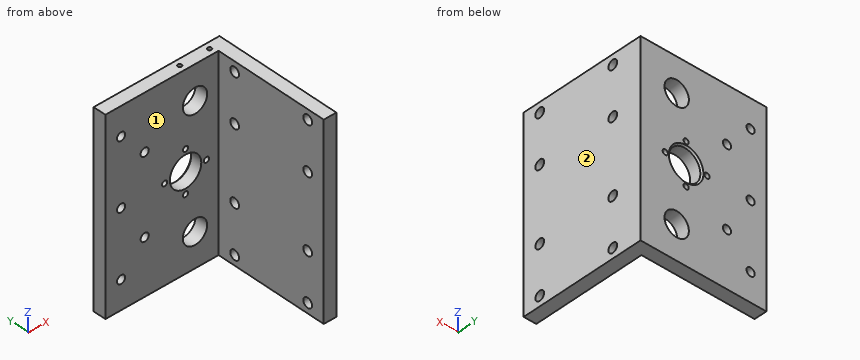
from build123d import *

# Parameters (mm, degrees)
ESTRUSIONE_ESTRUSIONE1_DEPTH = 120
TAGLIO_ESTRUSIONE2_REACH     = 82
SCHIZZO6_R                   = 7.75
TAGLIO_ESTRUSIONE3_REACH     = 82
SCHIZZO7_R                   = 10
M4_TAPPED_HOLE1_D            = 3.3
SCHIZZO12_R                  = 3
TAGLIO_ESTRUSIONE4_DEPTH     = 10
SCHIZZO14_R                  = 2.6
TAGLIO_ESTRUSIONE5_DEPTH     = 10
SMUSSO2_SIZE                 = 1
FORO_FILETTATO_M3_1_D        = 2.5
FORO_FILETTATO_M3_1_DEPTH    = 10
FORO_FILETTATO_M3_1_TIP      = 0.751075774


with BuildPart() as part:
    # Schizzo1 → Estrusione-Estrusione1 (new body)
    with BuildSketch(Plane.XY):
        Polygon((0, 0), (-80, 0), (-80, -8), (-8, -8), (-8, -80), (0, -80), align=None)
    extrude(amount=ESTRUSIONE_ESTRUSIONE1_DEPTH)

    # Schizzo6 → Taglio-Estrusione2 (cut, up to next)
    with BuildSketch(Plane(origin=(0, 0, 0), x_dir=(1, 0, 0), z_dir=(0, 1, 0)), mode=Mode.PRIVATE) as taglio_estrusione2_sk1:
        with Locations((-23, -21.5)):
            Circle(SCHIZZO6_R)
    taglio_estrusione2_tool1 = extrude(taglio_estrusione2_sk1.sketch, amount=-TAGLIO_ESTRUSIONE2_REACH, mode=Mode.PRIVATE) & part.part
    add(taglio_estrusione2_tool1.solids().sort_by_distance((-23, 0, 21.5))[0], mode=Mode.SUBTRACT)
    # Schizzo6 → Taglio-Estrusione2 (cut, up to next)
    with BuildSketch(Plane(origin=(0, 0, 0), x_dir=(1, 0, 0), z_dir=(0, 1, 0)), mode=Mode.PRIVATE) as taglio_estrusione2_sk2:
        with Locations((-23, -98.5)):
            Circle(SCHIZZO6_R)
    taglio_estrusione2_tool2 = extrude(taglio_estrusione2_sk2.sketch, amount=-TAGLIO_ESTRUSIONE2_REACH, mode=Mode.PRIVATE) & part.part
    add(taglio_estrusione2_tool2.solids().sort_by_distance((-23, 0, 98.5))[0], mode=Mode.SUBTRACT)

    # Schizzo7 → Taglio-Estrusione3 (cut, up to next)
    with BuildSketch(Plane(origin=(0, 0, 0), x_dir=(1, 0, 0), z_dir=(0, 1, 0)), mode=Mode.PRIVATE) as taglio_estrusione3_sk1:
        with Locations((-29, -60)):
            Circle(SCHIZZO7_R)
    taglio_estrusione3_tool1 = extrude(taglio_estrusione3_sk1.sketch, amount=-TAGLIO_ESTRUSIONE3_REACH, mode=Mode.PRIVATE) & part.part
    add(taglio_estrusione3_tool1.solids().sort_by_distance((-29, 0, 60))[0], mode=Mode.SUBTRACT)

    # M4 Tapped Hole1 (through all)
    with Locations(Plane(origin=(0, 0, 0), x_dir=(1, 0, 0), z_dir=(0, 1, 0))):
        with Locations((-29, -46.7), (-42.3, -60), (-29, -73.3), (-15.7, -60), (-29, -60)):
            Hole(M4_TAPPED_HOLE1_D / 2)

    # Schizzo12 → Taglio-Estrusione4 (cut)
    with BuildSketch(Plane(origin=(0, 0, 0), x_dir=(0, 0, -1), z_dir=(1, 0, 0))):
        with Locations((-113.75, -19)):
            Circle(SCHIZZO12_R)
        with Locations((-83.25, -19)):
            Circle(SCHIZZO12_R)
        with Locations((-36.75, -19)):
            Circle(SCHIZZO12_R)
        with Locations((-6.25, -19)):
            Circle(SCHIZZO12_R)
        with Locations((-83.25, -69)):
            Circle(SCHIZZO12_R)
        with Locations((-113.75, -69)):
            Circle(SCHIZZO12_R)
        with Locations((-6.25, -69)):
            Circle(SCHIZZO12_R)
        with Locations((-36.75, -69)):
            Circle(SCHIZZO12_R)
    extrude(amount=-TAGLIO_ESTRUSIONE4_DEPTH, mode=Mode.SUBTRACT)

    # Schizzo14 → Taglio-Estrusione5 (cut)
    with BuildSketch(Plane(origin=(0, 0, 0), x_dir=(1, 0, 0), z_dir=(0, 1, 0))):
        with Locations((-70, -18)):
            Circle(SCHIZZO14_R)
        with Locations((-70, -60)):
            Circle(SCHIZZO14_R)
        with Locations((-70, -102)):
            Circle(SCHIZZO14_R)
        with Locations((-55, -35)):
            Circle(SCHIZZO14_R)
        with Locations((-55, -85)):
            Circle(SCHIZZO14_R)
    extrude(amount=-TAGLIO_ESTRUSIONE5_DEPTH, mode=Mode.SUBTRACT)

    # Smusso2
    smusso2_edges = [part.edges().sort_by_distance(p)[0] for p in [
        (-39, 0, 60),
    ]]
    chamfer(smusso2_edges, length=SMUSSO2_SIZE)

    # Foro filettato M3-1
    with Locations(Plane.XY.offset(120)):
        with Locations((-10, -4), (-29, -4)):
            Hole(FORO_FILETTATO_M3_1_D / 2, depth=FORO_FILETTATO_M3_1_DEPTH)
            with Locations((0, 0, -(FORO_FILETTATO_M3_1_DEPTH + FORO_FILETTATO_M3_1_TIP / 2))):  # 118° drill point
                Cone(0, FORO_FILETTATO_M3_1_D / 2, FORO_FILETTATO_M3_1_TIP, mode=Mode.SUBTRACT)


solid = part.part
Check sheet for the modelled part. Datum: model origin and axes. Units: mm. Face numbers are marked on the shaded views. A direction names the side the tool comes from. Round coordinates to 2 decimals unless told otherwise and drop trailing zeros. Loops run counter-clockwise (first coordinate to the right, second up) from the corner with the lowest first, then second, coordinate; pieces in that order, holes last. Notation, with made-up numbers: (2, 71) -> (45, 71) arc R4 ccw to (45, 75) -> close; hole circle Ø1 at (77, -35). An arc over 180 degrees is marked (long way). Put each result on its own line as item: value. Start each with the question number.
1. Gauge pin test, flat ends, axial feed: pin 1 (3 mm diameter, centred on x = -55, z = 35, fed in from -Y); pin 2 (8 mm diameter, centred on y = -36.5, z = 100, fed in from -X); pin 3 (8.5 mm diameter, centred on x = -70, z = 18, fed in from -Y). Record the tip position at first contact, or that the pin passes through.
2. Scan lines: probe 1 along Z at (x, y) = (-55, -5); probe 2 along X at (y, z) = (-4, 60); probe 3 along Y at (x, z) = (-4, 83). Record each from-to range of solid material in increasing order.
3. Section check B-B (y = -69). Enter the section's corners in (x, z).
4. Section check D-D (x = -23). Give the number of separate pieces and of enclosed holes in the cut face, plus the area to 3 significant figures.
5. Section check A-A (z = 113.75). Enter the section's corners in (x, y).
6. Access from +Z, -Z, +X, -X, +Y, -Y to the whole of each face (thin tool, end or side, straight path). Record for the marked faces 1 and 2.
7. Section check C-C (z = 46.7). Enter the section's corners in (x, y).
Findings:
1. pin 1: passes through
1. pin 2: stops at x = -8
1. pin 3: stops at y = -8
2. probe 1: z = 0 to 32.4, 37.6 to 82.4, 87.6 to 120
2. probe 2: x = -80 to -72.6, -67.4 to -43.95, -40.65 to -39, -19 to -17.35, -14.05 to 0
2. probe 3: y = -80 to -71.99, -66.01 to -21.99, -16.01 to 0
3. outline: (-8, 0) -> (0, 0) -> (0, 3.25) -> (-8, 3.25) -> close; (-8, 9.25) -> (0, 9.25) -> (0, 33.75) -> (-8, 33.75) -> close; (-8, 39.75) -> (0, 39.75) -> (0, 80.25) -> (-8, 80.25) -> close; (-8, 86.25) -> (0, 86.25) -> (0, 110.75) -> (-8, 110.75) -> close; (-8, 116.75) -> (0, 116.75) -> (0, 120) -> (-8, 120) -> close
4. separate pieces: 4
4. enclosed holes: 0
4. area: 583 mm^2
5. outline: (-80, -8) -> (-8, -8) -> (-8, -16) -> (0, -16) -> (0, 0) -> (-80, 0) -> close; (-8, -80) -> (0, -80) -> (0, -72) -> (-8, -72) -> close; (-8, -66) -> (0, -66) -> (0, -22) -> (-8, -22) -> close; hole circle Ø2.5 at (-29, -4); hole circle Ø2.5 at (-10, -4)
6. face 1: +Z, -Z, -X, -Y
6. face 2: +Z, -Z, +X, +Y, -Y
7. outline: (-80, -8) -> (-30.65, -8) -> (-30.65, 0) -> (-80, 0) -> close; (-27.35, -8) -> (-8, -8) -> (-8, -80) -> (0, -80) -> (0, 0) -> (-27.35, 0) -> close
